Source: CAD feature listing. Evaluate the final solid. Frame: model axes, mm. A direction names the side the tool comes from. Round coordinates to 2 decimals unless told otherwise and drop trailing zeros. Loops run counter-clockwise (first coordinate to the right, second up) from the corner with the lowest first, then second, coordinate; pieces in that order, holes last.
(1) Set-up query: faces 1 (the cylindrical face through (5.9, -41.86, -3.07)), 2 (the flat face through (-3, -50.8, -3)), 3 (the flat face through (-2, 0, -2)). Return all of +Z, -Z, +X, -X, +Y, -Y with unobstructed straight access to the full face (end or side cutting, diameter ignored); none if empty.
(2) Section B-B, the plane x = 0. Return the cut outline in (y, z) (3 decimals).
(3) Section C-C, the plane y = -39. Return the cut outline in (x, z), plus the area to 3 significant figures.
(4) Material intervals for probe 1 along Y at (x, z) = (2.75, -3); probe 2 along Y at (x, z) = (-5, -1.25); probe 3 along Z at (x, y) = (4, -48), sorted ascending.
(5) Section A-A, the plane z = 0. Return the cut outline in (x, y) (3 decimals).
(6) First-contact query: pin 1 Ø1 at (y, z) = (-38, 4) entering from +X; pin 2 Ø6 at (x, y) = (-3.5, -10) entering from +Z; pin 3 Ø2 at (x, y) = (4, -5.5) entering from +Z. Flat tips, straight axial feed; report the tip coordinate or a pass-through.
(7) Section D-D, the plane y = -25. Return the cut outline in (x, z).
Autodesk Inventor part; units mm, degrees
ref_plane "YZ Plane" through (0, 0, 0) normal (1, 0, 0) x (0, 1, 0)
ref_plane "XZ Plane" through (0, 0, 0) normal (0, 1, 0) x (-1, 0, 0)
ref_plane "XY Plane" through (0, 0, 0) normal (0, 0, 1) x (1, 0, 0)
sketch "Sketch1" plane through (0, 0, 0) normal (1, 0, 0) x (0, 1, 0)
  line L0 (0, 0) -> (-9.3, 0)
  line L1 (-9.3, 0) -> (-9.3, -4.725)
  line L2 (-9.3, -4.725) -> (0, -4.725)
  line L3 (0, -4.725) -> (0, 0)
  line L4 (0, 0) -> (5, 0)
  line L5 (5, 0) -> (5, -2.5)
  line L6 (5, -2.5) -> (0, -2.5)
  line L7 (0, -2.5) -> (0, 0)
  line L8 (-9.3, 0) -> (-24.3, 0)
  line L9 (-24.3, 0) -> (-24.3, -5.27)
  line L10 (-24.3, -5.27) -> (-9.3, -5.27)
  line L11 (-9.3, -5.27) -> (-9.3, 0)
  line L12 (-24.3, 0) -> (-50.8, 0)
  line L13 (-50.8, 0) -> (-50.8, -6.65)
  line L14 (-50.8, -6.65) -> (-24.3, -6.65)
  line L15 (-24.3, -5.8531) -> (-24.3, 0)
  line L16 (-50.8, 0) -> (-54.4, 0)
  line L17 (-54.4, 0) -> (-54.4, -4)
  line L18 (-54.4, -4) -> (-50.8, -4)
  line L19 (-50.8, -4) -> (-50.8, 0)
  line L20 (-24.3, -5.8531) -> (-33.1623, -6.65)
  dimension "d0" = 9.3
  dimension "d1" = 4.725
  dimension "d2" = 5
  dimension "d3" = 2.5
  dimension "d4" = 15
  dimension "d5" = 26.5
  dimension "d6" = 6.65
  dimension "d7" = 5.27
  dimension "d8" = 3.6
  dimension "d9" = 4
revolve "Revolution1" add sketch "Sketch1" angle 360 about axis through (0, -9.3, 0) along (0, -1, 0)
properties part number "00_micrometer_xy-stage"
Output values:
1. face 1: +Y, -Y
1. face 2: -Y
1. face 3: +Y
2. outline: (-54.4, -4) - (-50.8, -4) - (-50.8, -6.65) - (-33.162, -6.65) - (-24.3, -5.853) - (-24.3, -5.27) - (-9.3, -5.27) - (-9.3, -4.725) - (0, -4.725) - (0, -2.5) - (5, -2.5) - (5, 2.5) - (0, 2.5) - (0, 4.725) - (-9.3, 4.725) - (-9.3, 5.27) - (-24.3, 5.27) - (-24.3, 5.853) - (-33.162, 6.65) - (-50.8, 6.65) - (-50.8, 4) - (-54.4, 4) - close
3. outline: circle Ø13.3 at (0, 0)
3. area: 139 mm2
4. probe 1: y = -50.8 to 0
4. probe 2: y = -50.8 to -9.3
4. probe 3: z = -5.31 to 5.31
5. outline: (-6.65, -50.8) - (-4, -50.8) - (-4, -54.4) - (4, -54.4) - (4, -50.8) - (6.65, -50.8) - (6.65, -33.162) - (5.853, -24.3) - (5.27, -24.3) - (5.27, -9.3) - (4.725, -9.3) - (4.725, 0) - (2.5, 0) - (2.5, 5) - (-2.5, 5) - (-2.5, 0) - (-4.725, 0) - (-4.725, -9.3) - (-5.27, -9.3) - (-5.27, -24.3) - (-5.853, -24.3) - (-6.65, -33.162) - close
6. pin 1: stops at x = 5.65
6. pin 2: stops at z = 5.25
6. pin 3: stops at z = 3.65
7. outline: circle Ø11.83 at (0, 0)
